Could you check a few things on this model? Use its own coordinates, in mm. Coordinates: 2 decimals unless noted, no trailing zeros. Order: outer loops, then holes, each group sorted by start corner. A loop starts at its lowest first (then second) coordinate and runs counter-clockwise, first axis right, second up. Notation, with made-up numbers: (-12.5, 51.25) -> (35.5, 51.25) arc R11 cw to (35.5, 64.25) -> close; hole circle Ø2 at (50.25, 11.25). An arc over 180 degrees is marked (long way). Put each result on its own line as item: value. Start each with the question number.
Q1. Will these pins go through, and if not, where does the flat tip stop? pin 1 (8 mm diameter, centred on y = 15.5, z = 1, fed in from -X); pin 2 (2 mm diameter, centred on y = 3.5, z = 9.5, fed in from +X); pin 3 (5 mm diameter, centred on x = 25, y = 5.5, fed in from -Z); pin 4 (1 mm diameter, centred on x = 2, y = 5, fed in from +Z).
Q2. If we section it at B-B (z = 9): Please give me the cut outline in (x, y), and give its area (3 significant figures).
Q3. Please list where these lines run through material, in increasing order: line 1 along X through (y, z) = (10.75, 0); line 2 along X through (y, z) = (6.5, 2.5); line 3 along Z through (x, y) = (0, 11.25).
Q4. We'd pull the mould along Z, two halves only. Please class faces 1 (the face through (30.5, 8.4, 12.6)), 2 (the face through (22, 0, 0)), 3 (the face through (14.49, 8.38, -26.53)): +Z half, -Z half, draft (parallel to the pull), parting line (faces both ways), or undercut.
Q5. If we section it at A-A (x = 0): Please give me the cut outline in (y, z).
Q6. If we section it at D-D (z = -24): Please give me the cut outline in (x, y).
Q7. If we section it at C-C (x = 13.5): Please give me the cut outline in (y, z).
from build123d import *

# Parameters (mm, degrees)
SKETCH1_R                = 33
SKETCH1_R_2              = 21
BOSS_EXTRUDE1_DEPTH      = 17
M6_CLEARANCE_HOLE1_D     = 6.6
M6_CLEARANCE_HOLE1_DEPTH = 17
CIRPATTERN1_COUNT        = 6


with BuildPart() as part:
    # Sketch1 → Boss-Extrude1 (new body)
    with BuildSketch(Plane(origin=(0, 0, 0), x_dir=(1, 0, 0), z_dir=(0, 1, 0))):
        Circle(SKETCH1_R)
        Circle(SKETCH1_R_2, mode=Mode.SUBTRACT)
    extrude(amount=BOSS_EXTRUDE1_DEPTH)

    # M6 Clearance Hole1
    with Locations(Plane(origin=(-27, 17, 0), x_dir=(0, 0, 1), z_dir=(0, 1, 0))):
        with Locations((0, 0)):
            m6_clearance_hole1 = Hole(M6_CLEARANCE_HOLE1_D / 2, depth=M6_CLEARANCE_HOLE1_DEPTH)

    # CirPattern1: M6 Clearance Hole1 ×6 about axis
    cirpattern1_axis = Axis((0, 0, 0), (0, 1, 0))
    for i in range(1, CIRPATTERN1_COUNT):
        add(m6_clearance_hole1.rotate(cirpattern1_axis, i * 360 / CIRPATTERN1_COUNT), mode=Mode.SUBTRACT)


solid = part.part
The answers:
1. pin 1: x = -33
1. pin 2: x = 31.89
1. pin 3: z = -24.14
1. pin 4: z = 32.97
2. outline: (-31.75, 0) -> (-18.97, 0) -> (-18.97, 17) -> (-31.75, 17) -> close; (18.97, 0) -> (31.75, 0) -> (31.75, 17) -> (18.97, 17) -> close
2. area: 434 mm^2
3. line 1: -33 to -30.3, -23.7 to -21, 21 to 23.7, 30.3 to 33
3. line 2: -32.91 to -29.15, -24.85 to -20.85, 20.85 to 24.85, 29.15 to 32.91
3. line 3: -33 to -21, 21 to 33
4. face 1: parting line
4. face 2: draft
4. face 3: undercut
5. outline: (0, -33) -> (17, -33) -> (17, -21) -> (0, -21) -> close; (0, 21) -> (17, 21) -> (17, 33) -> (0, 33) -> close
6. outline: (-22.65, 0) -> (-16.74, 0) -> (-16.74, 17) -> (-22.65, 17) -> close; (-10.26, 0) -> (10.26, 0) -> (10.26, 17) -> (-10.26, 17) -> close; (16.74, 0) -> (22.65, 0) -> (22.65, 17) -> (16.74, 17) -> close
7. outline: (0, -30.11) -> (17, -30.11) -> (17, -26.68) -> (0, -26.68) -> close; (0, -20.08) -> (17, -20.08) -> (17, -16.09) -> (0, -16.09) -> close; (0, 16.09) -> (17, 16.09) -> (17, 20.08) -> (0, 20.08) -> close; (0, 26.68) -> (17, 26.68) -> (17, 30.11) -> (0, 30.11) -> close
